Autodesk Inventor part; units mm, degrees
ref_plane "YZ Plane" through (0, 0, 0) normal (1, 0, 0) x (0, 1, 0)
ref_plane "XZ Plane" through (0, 0, 0) normal (0, 1, 0) x (-1, 0, 0)
ref_plane "XY Plane" through (0, 0, 0) normal (0, 0, 1) x (1, 0, 0)
sketch "Sketch1" plane through (0, 0, 0) normal (0, 1, 0) x (-1, 0, 0)
  line L0 (15, 7.5) -> (-15, 7.5)
  line L1 (-15, 7.5) -> (-15, -7.5)
  line L2 (-15, -7.5) -> (15, -7.5)
  line L3 (15, -7.5) -> (15, 7.5)
  line L4 (15, 7.5) -> (-15, -7.5) construction
  line L5 (-15, 7.5) -> (15, -7.5) construction
  line L6 (15, 7.5) -> (13, 7.5)
  line L7 (13, 7.5) -> (13, -7.5)
  line L8 (13, -7.5) -> (15, -7.5)
  line L9 (15, -7.5) -> (15, 7.5)
  circle A0 centre (6, 0) radius 1.5
  circle A1 centre (6, 0) radius 2.75
  line L10 (0, 7.5) -> (0, -7.5) construction
  circle A2 centre (-6, 0) radius 1.5
  circle A3 centre (-6, 0) radius 2.75
  point P0 (0, 0)
  dimension "d0" = 30
  dimension "d1" = 15
  dimension "d2" = 2
  dimension "d3" = 3
  dimension "d4" = 5.5
  dimension "d5" = 6
extrude "Extrusion1" add sketch "Sketch1" along normal blind 2 contours L7 L2 L1 L0
extrude "Extrusion2" add sketch "Sketch1" along normal blind 1 contours A1 | A3
extrude "Extrusion3" add sketch "Sketch1" along normal blind 29 contours L3 L2 L7 L0
sketch "Sketch2" plane through (-13, 2, -7.5) normal (1, 0, 0) x (0, 0, -1)
  line L0 (-15, 0) -> (-15, 27)
  circle A0 centre (-15, 12.25) radius 12.25
  line L1 (-15, 0) -> (0, 0)
  point P0 (-7.5, -2)
  point P1 (-15, 24.5)
  dimension "d15" = 24.5
  dimension "d16" = 12.25
extrude "Extrusion4" cut sketch "Sketch2" against normal blind 30 contours L0 A0 picked at (-11.8075, 14.7959)
sketch "Sketch3" plane through (-13, 2, -7.5) normal (1, 0, 0) x (0, 0, -1)
  line L0 (-15, 27) -> (0, 27)
  line L1 (-15, 27) -> (0, 27)
  line L2 (0, -2) -> (0, 0)
  line L3 (0, 27) -> (0, 0)
  line L4 (0, 0) -> (-15, 0)
  line L5 (0, 0) -> (-15, 0)
  arc A0 (-15, 0) -> (-15, 24.5) centre (-15, 12.25) ccw
  arc A1 (-15, 24.5) -> (-2.75, 12.25) centre (-15, 12.25) ccw
  line L6 (-15, 27) -> (-15, 24.5)
  line L7 (-15, 0) -> (-15, 24.5)
  point P0 (-7.5, -2)
extrude "Extrusion5" add sketch "Sketch3" along normal blind 3 contours L0 L3 L4 A0 L6
properties part number "Bracket Motor JGA Kanan_3DPrint"
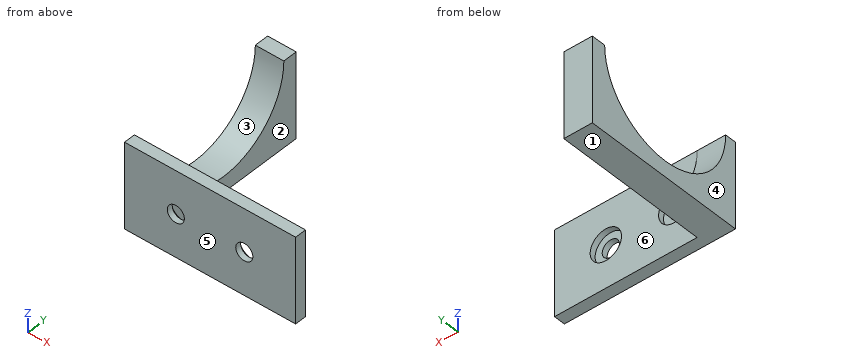
Could you check a few things on this model? Use its own coordinates, in mm. Face numbers are marked on the shaded views. A direction names the side the tool comes from. Coordinates: 2 decimals unless noted, no trailing zeros. Order: outer loops, then holes, each group sorted by start corner. A loop starts at its lowest first (then second) coordinate and runs counter-clockwise, first axis right, second up. Notation, with made-up numbers: (-32.5, -27.5) -> (-18.5, -27.5) arc R17 cw to (-18.5, -12.5) -> close; hole circle Ø8 at (26.25, -27.5). An arc over 180 degrees is marked (long way). One line per question, with ' | ' between items.
Q1. Imagine slicing it at D-D on y = 14.25. Please give me the cut outline in (x, z).
Return value:
outline: (-15, -7.5) -> (-10, -7.5) -> (-10, -4.75) -> (-15, -4.75) -> close
Q2. Imagine slicing it at C-C on x = -10.5. Please give me the cut outline in (y, z), and give its area (3 significant figures).
Return value:
outline: (0, -7.5) -> (29, -7.5) -> (29, 7.5) -> (26.5, 7.5) arc R12.25 cw to (2, 7.5) -> (0, 7.5) -> close | area: 199 mm²
Q3. If I drill on L1, parallel to Z at x = 6, y = 1.5; L2, parallel to Z at x = -6, y = 0.55; L3, parallel to Y at x = 11, z = -0.75, over which ranges is the centre line in solid material (lowest first)?
Return value:
L1: -7.5 to -2.75, 2.75 to 7.5 | L2: -7.5 to -1.5, 1.5 to 7.5 | L3: 0 to 2
Q4. Imagine slicing it at A-A on x = -6. Please give me the cut outline in (y, z), and give its area (3 significant figures).
Return value:
outline: (0, -7.5) -> (2, -7.5) -> (2, -2.75) -> (1, -2.75) -> (1, -1.5) -> (0, -1.5) -> close; (0, 1.5) -> (1, 1.5) -> (1, 2.75) -> (2, 2.75) -> (2, 7.5) -> (0, 7.5) -> close | area: 21.5 mm²
Q5. Thinking about a two-plate mould opening in Y: for the marked faces 3, 4, 5 and 6, which applies, pulls with the +Y half, pulls with the -Y half, needs draft (parallel to the pull), parting line crosses it, or undercut?
Return value:
face 3: undercut | face 4: needs draft | face 5: pulls with the -Y half | face 6: pulls with the +Y half
Q6. On a 3-axis mill with a long thin cutter (end or side, diameter ignored), from which of +Z, -Z, +X, -X, +Y, -Y can I reach the whole of each face in a straight line? I mean the marked faces 1 and 2. Say none if no direction works.
Return value:
face 1: -Z, +X, -X, +Y, -Y | face 2: +Z, -Z, +X, +Y
Q7. Imagine slicing it at B-B on z = 0. Please give me the cut outline in (x, y), and give its area (3 significant figures).
Return value:
outline: (-15, 0) -> (-7.5, 0) -> (-7.5, 1) -> (-8.75, 1) -> (-8.75, 2) -> (-10, 2) -> (-10, 4.56) -> (-15, 4.56) -> close; (-15, 23.94) -> (-10, 23.94) -> (-10, 29) -> (-15, 29) -> close; (-4.5, 0) -> (4.5, 0) -> (4.5, 1) -> (3.25, 1) -> (3.25, 2) -> (-3.25, 2) -> (-3.25, 1) -> (-4.5, 1) -> close; (7.5, 0) -> (15, 0) -> (15, 2) -> (8.75, 2) -> (8.75, 1) -> (7.5, 1) -> close | area: 81.1 mm²
Q8. I'm going to push flat-ended pins straight in: P1, Ø6, axis at x = 5.5, z = -1.5, coming from the +Y side; P2, Ø5, axis at x = -6, z = 0, coming from the +Y side; P3, Ø3, axis at y = 17, z = -2, coming from the -X side. Where does each tip first touch, or does it pass through?
Return value:
P1: y = 2 | P2: y = 1 | P3: through
